The drawing under review shows one solid part. Ordinate dimensions are in mm from its lowest x, y, z. Coordinates: 2 decimals unless noted, no trailing zeros.
1) Insertion check: P1, Ø3, axis at x = 2.5, z = 2.5, coming from the +Y side; P2, Ø4, axis at x = 48, z = 10.5, coming from the -Y side. Each pin has a flat end and moves straight along its axis. Give the tip position at first contact, or say it passes through.
2) Mouldability with a two-part tool opening along Y and no side actions: class the marked faces 1 and 2 as pulls with the +Y half, pulls with the -Y half, needs draft (parallel to the pull), parting line crosses it, or undercut.
3) To check wall thickness, follow line 1 along X through (y, z) = (0.65, 2.5); line 2 along Z through (x, y) = (2.5, 0.5). State the ranges of each line that lie inside material, in increasing order.
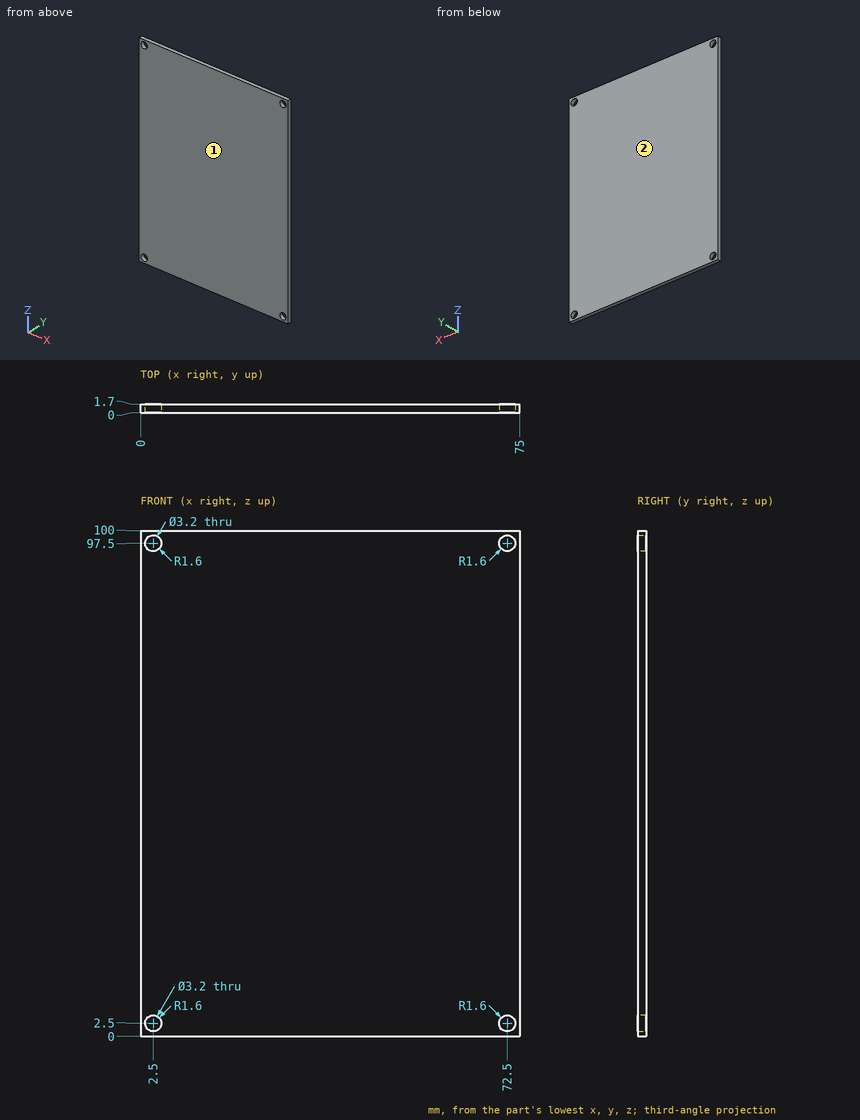
Result:
1. P1: passes through
1. P2: stops at y = 0
2. face 1: pulls with the -Y half
2. face 2: pulls with the +Y half
3. line 1: x = 0 to 0.9, 4.1 to 70.9, 74.1 to 75
3. line 2: z = 0 to 0.9, 4.1 to 95.9, 99.1 to 100
